Autodesk Inventor part; units mm, degrees
ref_plane "YZ Plane" through (0, 0, 0) normal (1, 0, 0) x (0, 1, 0)
ref_plane "XZ Plane" through (0, 0, 0) normal (0, 1, 0) x (-1, 0, 0)
ref_plane "XY Plane" through (0, 0, 0) normal (0, 0, 1) x (1, 0, 0)
sketch "Boceto1" plane through (0, 0, 0) normal (0, 0, 1) x (1, 0, 0)
  circle A0 centre (0, 0) radius 115
  line L0 (105, 0) -> (105, 65)
  line L1 (105, 65) -> (105, -65)
  line L2 (105, -65) -> (85, -65)
  line L3 (85, -65) -> (85, 65)
  line L4 (85, 65) -> (105, 65)
  line L5 (-105, 0) -> (-105, 65)
  line L6 (-105, 65) -> (-85, 65)
  line L7 (-85, 65) -> (-85, -65)
  line L8 (-85, -65) -> (-105, -65)
  line L9 (-105, -65) -> (-105, 0)
  dimension "d0" = 230
  dimension "d33" = 65
  dimension "d34" = 130
  dimension "d35" = 20
  dimension "d36" = 65
  dimension "d37" = 20
extrude "Extrusión1" add sketch "Boceto1" along normal blind 10 contours A0 L1 L0 | L0 L1 A0 L2 L3 L4 | L4 L3 L2 A0 L8 L7 L6 | L6 L7 L8 A0 L9 L5 | L5 L9 A0
sketch "Boceto2" plane through (0, 0, 10) normal (0, 0, 1) x (1, 0, 0)
  circle A0 centre (0, 0) radius 17.5
  circle A1 centre (0, 0) radius 14.9
  dimension "d4" = 35
  dimension "d21" = 29.8
extrude "Extrusión2" add sketch "Boceto2" along normal blind 5 contours A0 | A1
sketch "Boceto3" plane through (0, 0, 15) normal (0, 0, 1) x (1, 0, 0)
  circle A0 centre (0, 0) radius 14.9
  dimension "d20" = 29.8
extrude "Extrusión3" [suppressed]
sketch "Boceto4" plane through (0, 0, 0) normal (0, 0, -1) x (-1, 0, 0)
  line L0 (105, 0) -> (-105, 0)
  line L1 (-105, 0) -> (-105, 65)
  line L2 (-105, 65) -> (-85, 65)
  line L3 (-85, 65) -> (-85, -65)
  line L4 (-85, -65) -> (-105, -65)
  line L5 (-105, -65) -> (-105, 0)
  line L6 (105, 0) -> (105, -65)
  line L7 (105, -65) -> (85, -65)
  line L8 (85, -65) -> (85, 65)
  line L9 (85, 65) -> (105, 65)
  line L10 (105, 65) -> (105, 0)
  point P0 (0, 0)
  dimension "d40" = 65
  dimension "d41" = 20
  dimension "d42" = 130
  dimension "d43" = 65
  dimension "d44" = 20
  dimension "d45" = 130
sketch "Boceto5" plane through (0, 0, 15) normal (0, 0, 1) x (1, 0, 0)
  circle A0 centre (0, 0) radius 14.9
  dimension "d22" = 29.8
extrude "Extrusión4" add sketch "Boceto5" along normal blind 10
ref_plane "Plano de trabajo2" through (0, 0, 5) normal (0, 0, -1) x (-1, 0, 0)
extrude "Extrusión5" cut sketch "Boceto4" against normal blind 5
properties part number "plato"
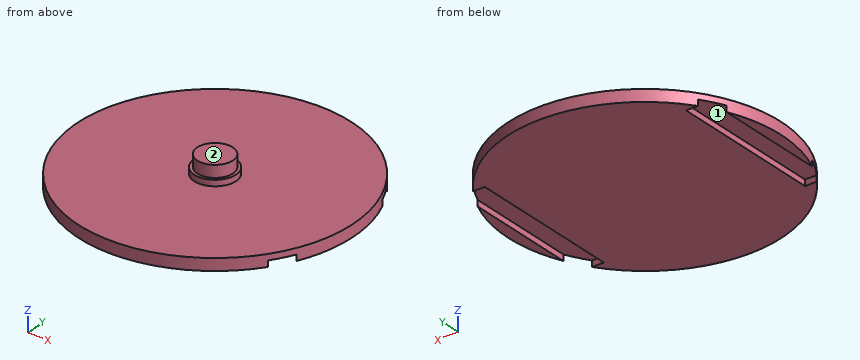
Geometry check sheet. Reference: the model listing, model coordinates, mm. Face numbers are marked on the shaded views. Coordinates: 2 decimals unless noted, no trailing zeros. Order: outer loops, then holes, each group sorted by start corner. A loop starts at its lowest first (then second) coordinate and runs counter-clockwise, first axis right, second up. Notation, with made-up numbers: (26, 89) - (56, 89) arc R28 cw to (56, 107) - close; hole circle Ø10 at (-26.5, 8.5). An arc over 180 degrees is marked (long way). One line per item, written item: value.
(1) Release check for a two-part mould opening along Y. For the marked faces 1 and 2 record: +Y half, -Y half, draft (parallel to the pull), parting line (faces both ways), or undercut.
Data:
face 1: undercut
face 2: draft
(2) Thickness scan on probe 1 along Z at (x, y) = (70, 3.5); probe 2 along X at (y, z) = (-40, 3.5); probe 3 along Y at (x, z) = (-81.5, 3). Record the ranges inside material, lowest first. Write a range as from..to.
Data:
probe 1: z = 0..10
probe 2: x = -107.82..-105, -85..85, 105..107.82
probe 3: y = -81.13..81.13
(3) Sectioned sample at C-C (z = 20). Enter the section's corners in (x, y).
Data:
outline: circle Ø29.8 at (0, 0)
(4) Sectioned sample at D-D (y = 28). Enter the section's corners in (x, z).
Data:
outline: (-111.54, 0) - (-105, 0) - (-105, 5) - (-85, 5) - (-85, 0) - (85, 0) - (85, 5) - (105, 5) - (105, 0) - (111.54, 0) - (111.54, 10) - (-111.54, 10) - close
(5) Sectioned sample at A-A (y = 0). Enter the section's corners in (x, z), and give its area (3 significant figures).
Data:
outline: (-115, 0) - (-105, 0) - (-105, 5) - (-85, 5) - (-85, 0) - (85, 0) - (85, 5) - (105, 5) - (105, 0) - (115, 0) - (115, 10) - (17.5, 10) - (17.5, 15) - (14.9, 15) - (14.9, 25) - (-14.9, 25) - (-14.9, 15) - (-17.5, 15) - (-17.5, 10) - (-115, 10) - close
area: 2,570 mm^2
(6) Sectioned sample at B-B (x = 0). Enter the section's corners in (y, z), and give its area (3 significant figures).
Data:
outline: (-115, 0) - (115, 0) - (115, 10) - (17.5, 10) - (17.5, 15) - (14.9, 15) - (14.9, 25) - (-14.9, 25) - (-14.9, 15) - (-17.5, 15) - (-17.5, 10) - (-115, 10) - close
area: 2,770 mm^2
(7) Depth check by flat-ended pin: pin 1 Ø12 at (x, z) = (-9, 4) entering from +Y; pin 2 Ø10 at (y, z) = (63, 17) entering from -X; pin 3 Ø16 at (x, y) = (-94.5, 32) entering from -Z; pin 4 Ø1.5 at (y, z) = (-21, 2.5) entering from +X. Enter the tip coordinate at first touch or a pass-through.
Data:
pin 1: stops at y = 114.96
pin 2: passes through
pin 3: stops at z = 5
pin 4: stops at x = 113.2
